Geometry: final body of the model. Coordinates: model frame, mm. A direction names the side the tool comes from. Give positions to 0.01 mm unless a question says otherwise; leave off trailing zeros. Write each loop counter-clockwise with the first axis right and the second up, starting at its lowest first coordinate (ties: lowest second). Pieces come first, ordered by that corner, then holes. Notation, with made-up numbers: M 47.5,46 L 106.5,46 A20 cw 106.5,60 Z; hole C 51.25,58.25 d10. An arc over 180 degrees is marked long. Answer as a JSON object with one key per item and string values.
from build123d import *

# Parameters (mm, degrees)
SKETCH2_W                    = 246.4
SKETCH2_H                    = 27.4
BASE_FLANGE2_DEPTH           = 0.8
EDGE_FLANGE1_STRIP_W         = 5.2
EDGE_FLANGE1_STRIP_H         = 0.8
EDGE_FLANGE1_STRIP_CUT_DEPTH = 27.4
EDGE_FLANGE1_DEPTH           = 27.4
EDGE_FLANGE2_STRIP_W         = 5.2
EDGE_FLANGE2_STRIP_H         = 0.8
EDGE_FLANGE2_STRIP_CUT_DEPTH = 27.4
EDGE_FLANGE2_DEPTH           = 27.4
EDGE_FLANGE3_STRIP_W         = 5.2
EDGE_FLANGE3_STRIP_H         = 0.8
EDGE_FLANGE3_STRIP_CUT_DEPTH = 244.4
EDGE_FLANGE3_DEPTH           = 244.4


# Sheet-metal steps are written as plain solids
with BuildPart() as part:
    # Sketch2 → Base-Flange2 (new body)
    with BuildSketch(Plane(origin=(0, 0, 0), x_dir=(0, 0, -1), z_dir=(1, 0, 0))):
        Rectangle(SKETCH2_W, SKETCH2_H)
    extrude(amount=BASE_FLANGE2_DEPTH)

    # Edge-Flange1 strip (across the edge) → Edge-Flange1 strip cut (cut)
    with BuildSketch(Plane(origin=(0.8, 13.7, 123.2), x_dir=(0, 0, -1), z_dir=(0, -1, 0))):
        with Locations((-1.6, -0.4)):
            Rectangle(EDGE_FLANGE1_STRIP_W, EDGE_FLANGE1_STRIP_H)
    extrude(amount=EDGE_FLANGE1_STRIP_CUT_DEPTH, mode=Mode.SUBTRACT)

    # Edge-Flange1 section (across the edge) → Edge-Flange1 (add)
    with BuildSketch(Plane(origin=(0.8, 13.7, 123.2), x_dir=(0, 0, -1), z_dir=(0, -1, 0))):
        with BuildLine():
            Line((-0.8, 1), (-0.8, 19.2))
            Line((-0.8, 19.2), (0, 19.2))
            Line((0, 19.2), (0, 1))
            ThreePointArc((0, 1), (0.292893219, 0.292893219), (1, 0))
            Line((1, 0), (1, -0.8))
            ThreePointArc((1, -0.8), (-0.272792206, -0.272792206), (-0.8, 1))
        make_face()
    extrude(amount=EDGE_FLANGE1_DEPTH)

    # Edge-Flange2 strip (across the edge) → Edge-Flange2 strip cut (cut)
    with BuildSketch(Plane(origin=(0.8, -13.7, -123.2), x_dir=(0, 0, 1), z_dir=(0, 1, 0))):
        with Locations((-1.6, -0.4)):
            Rectangle(EDGE_FLANGE2_STRIP_W, EDGE_FLANGE2_STRIP_H)
    extrude(amount=EDGE_FLANGE2_STRIP_CUT_DEPTH, mode=Mode.SUBTRACT)

    # Edge-Flange2 section (across the edge) → Edge-Flange2 (add)
    with BuildSketch(Plane(origin=(0.8, -13.7, -123.2), x_dir=(0, 0, 1), z_dir=(0, 1, 0))):
        with BuildLine():
            Line((-0.8, 1), (-0.8, 19.2))
            Line((-0.8, 19.2), (0, 19.2))
            Line((0, 19.2), (0, 1))
            ThreePointArc((0, 1), (0.292893219, 0.292893219), (1, 0))
            Line((1, 0), (1, -0.8))
            ThreePointArc((1, -0.8), (-0.272792206, -0.272792206), (-0.8, 1))
        make_face()
    extrude(amount=EDGE_FLANGE2_DEPTH)

    # Edge-Flange3 strip (across the edge) → Edge-Flange3 strip cut (cut)
    with BuildSketch(Plane(origin=(0.8, -13.7, 122.2), x_dir=(0, 1, 0), z_dir=(0, 0, -1))):
        with Locations((-1.6, -0.4)):
            Rectangle(EDGE_FLANGE3_STRIP_W, EDGE_FLANGE3_STRIP_H)
    extrude(amount=EDGE_FLANGE3_STRIP_CUT_DEPTH, mode=Mode.SUBTRACT)

    # Edge-Flange3 section (across the edge) → Edge-Flange3 (add)
    with BuildSketch(Plane(origin=(0.8, -13.7, 122.2), x_dir=(0, 1, 0), z_dir=(0, 0, -1))):
        with BuildLine():
            Line((-0.8, 1), (-0.8, 19.2))
            Line((-0.8, 19.2), (0, 19.2))
            Line((0, 19.2), (0, 1))
            ThreePointArc((0, 1), (0.292893219, 0.292893219), (1, 0))
            Line((1, 0), (1, -0.8))
            ThreePointArc((1, -0.8), (-0.272792206, -0.272792206), (-0.8, 1))
        make_face()
    extrude(amount=EDGE_FLANGE3_DEPTH)


solid = part.part
1) Contact query for flat-ended pins moving along their axis: P1, Ø1.4, axis at x = 6.5, z = -123, coming from the -Y side; P2, Ø13, axis at y = -2, z = -35.5, coming from the +X side. Output: stop coordinate, or through.
Geometry check:
{"P1": "stops at y = -13.7", "P2": "stops at x = 0.8"}
2) Pull-direction query (Z, two-part tool) for faces 4 (the flat face through (11, 0, -123.2)), 5 (the flat face through (11, 0, -124)), 6 (the flat face through (0.4, 13.7, 0.6)); classes: pulls with the +Z half, pulls with the -Z half, needs draft (parallel to the pull), parting line crosses it, or undercut.
Geometry check:
{"face 4": "undercut", "face 5": "pulls with the -Z half", "face 6": "needs draft"}
3) Cut plane B-B on z = 72. Return loops of the section in (x, y), and give its area (3 significant figures).
Geometry check:
{"outline": "M 0,-12.7 A1.8 ccw 1.8,-14.5 L 20,-14.5 L 20,-13.7 L 1.8,-13.7 A1 cw 0.8,-12.7 L 0.8,13.7 L 0,13.7 Z", "area": "37.4 mm2"}
4) Cut plane C-C on y = -3.75. Return loops of the section in (x, z).
Geometry check:
{"outline": "M 0,-122.2 A1.8 ccw 1.8,-124 L 20,-124 L 20,-123.2 L 1.8,-123.2 A1 cw 0.8,-122.2 L 0.8,122.2 A1 cw 1.8,123.2 L 20,123.2 L 20,124 L 1.8,124 A1.8 ccw 0,122.2 Z"}
5) Set-up query: faces 1 (the flat face through (0, 1, 2)), 2 (the flat face through (11, -13.7, 2)), 3 (the flat face through (11, 0, 123.2)). Return all of +Z, -Z, +X, -X, +Y, -Y with unobstructed straight access to the full face (end or side cutting, diameter ignored); none if empty.
Geometry check:
{"face 1": "+Z, -Z, -X, +Y, -Y", "face 2": "+X, +Y", "face 3": "+X, +Y, -Y"}
6) Line query: line 1 (Z direction, x = 2, y = 3); line 2 (Y direction, x = 2.5, z = -58.5); line 3 (X direction, y = 10.25, z = -24). Output: solid intervals per line, ascending. Write a range as from..to.
Geometry check:
{"line 1": "z = -124..-123.2, 123.2..124", "line 2": "y = -14.5..-13.7", "line 3": "x = 0..0.8"}
7) Cut plane A-A on x = 4. Return loops of the section in (y, z).
Geometry check:
{"outline": "M -14.5,-122.2 L -13.7,-122.2 L -13.7,122.2 L -14.5,122.2 Z; M -13.7,-124 L 13.7,-124 L 13.7,-123.2 L -13.7,-123.2 Z; M -13.7,123.2 L 13.7,123.2 L 13.7,124 L -13.7,124 Z"}
